Part model, mm, in its own coordinate system. A direction names the side the tool comes from. Round coordinates to 2 decimals unless told otherwise and drop trailing zeros. Loops run counter-clockwise (first coordinate to the right, second up) from the corner with the lowest first, then second, coordinate; pieces in that order, holes last. Notation, with made-up numbers: (-2.5, -27.5) -> (42.5, -27.5) arc R10 ccw to (42.5, -19.5) -> close; hole circle Ø9 at (20.25, 5.25). An arc over 180 degrees is marked (long way). Use a Markdown table: item, result. Add a question column.
Item 1: Two-plate mould, pull along X, no slides. Class faces 4 (the face through (-28, -3, -55)), 5 (the face through (-57, 2, -46)), 6 (the face through (-42.453, 0.409, -61.585)), 7 (the face through (-49.016, 0.409, -4.133)): pulls with the +X half, pulls with the -X half, needs draft (parallel to the pull), parting line crosses it, or undercut.
Item 2: Probe line 1 (X direction, y = 5.1, z = -66); line 2 (X direction, y = 0.75, z = -4) (3 decimals); line 3 (X direction, y = 1, z = -60). List the from-to ranges inside material, lowest first. Write a range as [from, to].
Item 3: Which spindle directions (+Z, -Z, +X, -X, +Y, -Y) get a long thin tool onto all of the face, cutting with end or side? Do faces 1 (the face through (-29, -3, -64)), 2 (the face through (-42.42, 3.96, -66.75)), 3 (the face through (-28, -3, -9)). Say none if no direction does.
Item 4: Cut at A-A, the plane y = -2.5. List the corners of the cut face in (x, z) (3 decimals).
Item 5: Cut at D-D, the plane z = -66. List the corners of the cut face in (x, y).
Item 6: Cut at B-B, the plane z = -4. List the corners of the cut face in (x, y) (3 decimals).
Item 7: Cut at C-C, the plane x = -15. List the corners of the cut face in (y, z).
Item 8: Flat gauge pins, fed straight in: pin 1 (3.5 mm diameter, centred on x = -37, y = -2.5, fed in from -Z); pin 2 (8.5 mm diameter, centred on x = -25, z = -84.5, fed in from -Y); pin 3 (3.5 mm diameter, centred on x = -15, z = -60, fed in from +Y); pin 4 (4 mm diameter, centred on x = -29.5, z = -19.5, fed in from -Y). Where does each tip first touch, or does it go through?
Autodesk Inventor part; units mm, degrees
ref_plane "YZ Plane" through (0, 0, 0) normal (1, 0, 0) x (0, 1, 0)
ref_plane "XZ Plane" through (0, 0, 0) normal (0, 1, 0) x (-1, 0, 0)
ref_plane "XY Plane" through (0, 0, 0) normal (0, 0, 1) x (1, 0, 0)
sketch "Sketch1" plane through (0, 0, 0) normal (0, 1, 0) x (-1, 0, 0)
  line L0 (0, 0) -> (57, 0)
  line L1 (57, 0) -> (57, -64)
  line L2 (57, -64) -> (0, -64)
  line L3 (0, -64) -> (0, 0)
  dimension "d0" = 57
  dimension "d1" = 64
extrude "Extrusion1" add sketch "Sketch1" along normal blind 7
sketch "Sketch2" plane through (0, 7, 0) normal (0, 1, 0) x (1, 0, 0)
  line L0 (-57, 64) -> (-57, 0)
  line L1 (-57, 0) -> (0, 0)
  line L2 (0, 64) -> (-57, 64)
  point P0 (-41, 4)
  point P1 (-15, 4)
  point P2 (-41, 60)
  point P3 (-15, 60)
  dimension "d4" = 26
  dimension "d5" = 16
  dimension "d6" = 4
  dimension "d7" = 4
  dimension "d8" = 4
  dimension "d9" = 4
  dimension "d10" = 26
  dimension "d11" = 16
sketch "Sketch3" plane through (0, 0, 0) normal (0, -1, 0) x (1, 0, 0)
  line L0 (0, -64) -> (-57, -64)
  line L1 (0, 0) -> (0, -64)
  line L2 (-57, -64) -> (0, -64)
  line L3 (0, -64) -> (0, -55)
  line L4 (0, -55) -> (-57, -55)
  line L5 (-57, -55) -> (-57, -64)
  line L6 (-57, -64) -> (-57, 0)
  line L7 (-57, 0) -> (0, 0)
  line L8 (0, 0) -> (0, -9)
  line L9 (0, -9) -> (-57, -9)
  line L10 (-57, -9) -> (-57, 0)
  dimension "d12" = 9
  dimension "d13" = 9
extrude "Extrusion2" add sketch "Sketch3" along normal blind 6 contours L0 L5 L4 L1 | L9 L6 L7 L1
hole "Hole1" at (-41, 7, -4) at (-15, 7, -4) at (-41, 7, -60) at (-15, 7, -60) direction (0, -1, 0) diameter 4.3 end through all
sketch "Sketch4" plane through (0, 7, 0) normal (0, 1, 0) x (1, 0, 0)
  line L0 (-57, 0) -> (0, 0)
  line L1 (-57, 64) -> (-57, 0)
  line L2 (0, 0) -> (0, 64)
  line L3 (-63.6235, 34) -> (1.4941, 34) construction
  line L4 (-48, -4.864) -> (-48, 68.9429) construction
  point P0 (-48, 4)
  point P1 (-48, 34)
  point P2 (-18, 34)
  dimension "d28" = 4
  dimension "d30" = 9
  dimension "d41" = 30
  dimension "d42" = 30
hole "Hole2" at (-48, 7, -4) at (-48, 7, -34) at (-18, 7, -34) direction (0, -1, 0) diameter 2.05 end through all
sketch "Sketch5" plane through (0, 7, -64) normal (0, 0, -1) x (-1, 0, 0)
  line L0 (57, -13) -> (57, 0)
  line L1 (0, 0) -> (57, 0)
  line L2 (57, 0) -> (57, -6)
  line L3 (57, -6) -> (0, -6)
  line L4 (0, -6) -> (0, 0)
  point P0 (0, -7)
  dimension "d43" = 6
extrude "Extrusion3" add sketch "Sketch5" along normal blind 28.63
sketch "Sketch6" plane through (0, 7, 0) normal (0, 1, 0) x (1, 0, 0)
  line L0 (-43, 25.0666) -> (-43, 99.5095) construction
  line L1 (-57, 92.63) -> (0, 92.63)
  line L2 (-22, 34.9149) -> (-22, 94.8811) construction
  line L3 (-39.656, 66) -> (-5.0422, 66) construction
  line L4 (-57, 0) -> (0, 0)
  line L5 (0, 0) -> (0, 92.63)
  line L6 (-49.1509, 78.5) -> (-3.6175, 78.5) construction
  point P0 (-43, 66)
  point P1 (-22, 66)
  point P2 (-43, 78.5)
  point P3 (-22, 78.5)
  dimension "d46" = 21
  dimension "d47" = 66
  dimension "d48" = 22
  dimension "d49" = 12.5
hole "Hole3" at (-43, 7, -66) at (-22, 7, -66) at (-43, 7, -78.5) at (-22, 7, -78.5) direction (0, -1, 0) diameter 1.9 end through all
properties part number "P132SupportCamera"
A:
| question | item | result |
|---|---|---|
| 1 | face 4 | needs draft |
| 1 | face 5 | pulls with the -X half |
| 1 | face 6 | undercut |
| 1 | face 7 | undercut |
| 2 | line 1 | x = [-57, -43.95], [-42.05, -22.95], [-21.05, 0] |
| 2 | line 2 | x = [-57, -49.025], [-46.975, -43.15], [-38.85, -17.15], [-12.85, 0] |
| 2 | line 3 | x = [-57, -43.15], [-38.85, -17.15], [-12.85, 0] |
| 3 | face 1 | -Z, +X, -X, -Y |
| 3 | face 2 | +Y, -Y |
| 3 | face 3 | +X, -X, -Y |
| 4 | outline | (-57, -64) -> (0, -64) -> (0, -55) -> (-57, -55) -> close; (-57, -9) -> (0, -9) -> (0, 0) -> (-57, 0) -> close; hole circle Ø2.05 at (-48, -4); hole circle Ø4.3 at (-41, -60); hole circle Ø4.3 at (-41, -4); hole circle Ø4.3 at (-15, -60); hole circle Ø4.3 at (-15, -4) |
| 5 | outline | (-57, 1) -> (-43.95, 1) -> (-43.95, 7) -> (-57, 7) -> close; (-42.05, 1) -> (-22.95, 1) -> (-22.95, 7) -> (-42.05, 7) -> close; (-21.05, 1) -> (0, 1) -> (0, 7) -> (-21.05, 7) -> close |
| 6 | outline | (-57, -6) -> (-49.025, -6) -> (-49.025, 7) -> (-57, 7) -> close; (-46.975, -6) -> (-43.15, -6) -> (-43.15, 7) -> (-46.975, 7) -> close; (-38.85, -6) -> (-17.15, -6) -> (-17.15, 7) -> (-38.85, 7) -> close; (-12.85, -6) -> (0, -6) -> (0, 7) -> (-12.85, 7) -> close |
| 7 | outline | (-6, -64) -> (1, -64) -> (1, -92.63) -> (7, -92.63) -> (7, -62.15) -> (-6, -62.15) -> close; (-6, -57.85) -> (7, -57.85) -> (7, -6.15) -> (-6, -6.15) -> (-6, -9) -> (0, -9) -> (0, -55) -> (-6, -55) -> close; (-6, -1.85) -> (7, -1.85) -> (7, 0) -> (-6, 0) -> close |
| 8 | pin 1 | stops at z = -64 |
| 8 | pin 2 | stops at y = 1 |
| 8 | pin 3 | passes through |
| 8 | pin 4 | stops at y = 0 |
